from build123d import *

# Parameters (mm, degrees)
SKETCH3_W                      = 31.148374891
SKETCH3_H                      = 19.837641971
BOSS_EXTRUDE1_DEPTH            = 6.35
SKETCH4_R                      = 3.175
CUT_EXTRUDE1_DEPTH             = 9.525
SKETCH5_R                      = 3.175
CUT_EXTRUDE5_DEPTH             = 9.525
CUT_EXTRUDE5_DIRECTION_2_REACH = 33.299
SKETCH6_R                      = 3.175
CUT_EXTRUDE6_DEPTH             = 9.525
SKETCH8_W                      = 12.7
SKETCH8_H                      = 1.803641971
CUT_EXTRUDE7_DEPTH             = 38.470999417
SKETCH9_W                      = 1.905
SKETCH9_H                      = 18.034
BOSS_EXTRUDE2_DEPTH            = 4.7625
SKETCH11_W                     = 1.190625
SKETCH11_H                     = 1.906


with BuildPart() as part:
    # Sketch3 → Boss-Extrude1 (new, symmetric)
    with BuildSketch(Plane.XY):
        with Locations((15.574187446, -9.918820986)):
            Rectangle(SKETCH3_W, SKETCH3_H)
    extrude(amount=BOSS_EXTRUDE1_DEPTH, both=True)

    # Sketch4 → Cut-Extrude1 (cut)
    with BuildSketch(Plane.ZY):
        with Locations(Location((0, -6.35, 0), (0, 0, 270))):
            Circle(SKETCH4_R)
    cut_extrude1 = extrude(amount=-CUT_EXTRUDE1_DEPTH, mode=Mode.SUBTRACT)

    # Sketch5 → Cut-Extrude5 (cut)
    with BuildSketch(Plane(origin=(7.787093723, -19.837641971, 0), x_dir=(-0.8660254037844382, 0.500000000000001, 0), z_dir=(-0.500000000000001, -0.8660254037844382, 0))):
        with Locations(Location((0, 0, 0), (0, 0, 180))):
            Circle(SKETCH5_R)
    cut_extrude5 = extrude(amount=-CUT_EXTRUDE5_DEPTH, mode=Mode.SUBTRACT)

    # Sketch5 → Cut-Extrude5 direction 2 (cut, up to next)
    with BuildSketch(Plane(origin=(7.787093723, -19.837641971, 0), x_dir=(-0.8660254037844382, 0.500000000000001, 0), z_dir=(-0.500000000000001, -0.8660254037844382, 0)), mode=Mode.PRIVATE) as cut_extrude5_direction_2_sk1:
        with Locations(Location((0, 0, 0), (0, 0, 180))):
            Circle(SKETCH5_R)
    cut_extrude5_direction_2_tool1 = extrude(cut_extrude5_direction_2_sk1.sketch, amount=CUT_EXTRUDE5_DIRECTION_2_REACH, mode=Mode.PRIVATE) & part.part
    cut_extrude5_direction_2 = cut_extrude5_direction_2_tool1.solids().sort_by_distance((7.787094, -19.837642, 0))[0]
    add(cut_extrude5_direction_2, mode=Mode.SUBTRACT)

    # Sketch6 → Cut-Extrude6 (cut)
    with BuildSketch(Plane(origin=(0, 0, -6.35), x_dir=(-1, 0, 0), z_dir=(0, 0, -1))):
        with Locations((-15.574187445, -6.35)):
            Circle(SKETCH6_R)
    extrude(amount=-CUT_EXTRUDE6_DEPTH, mode=Mode.SUBTRACT)

    # Mirror1: Cut-Extrude1, Cut-Extrude5, Cut-Extrude5 direction 2 across plane
    add(cut_extrude1.mirror(Plane.ZY.offset(-15.574187445)), mode=Mode.SUBTRACT)
    add(cut_extrude5.mirror(Plane.ZY.offset(-15.574187445)), mode=Mode.SUBTRACT)
    add(cut_extrude5_direction_2.mirror(Plane.ZY.offset(-15.574187445)), mode=Mode.SUBTRACT)

    # Sketch8 → Cut-Extrude7 (cut, through all)
    with BuildSketch(Plane(origin=(31.148374891, 0, 0), x_dir=(0, 0, -1), z_dir=(1, 0, 0))):
        with Locations((0, -18.935820986)):
            Rectangle(SKETCH8_W, SKETCH8_H)
    extrude(amount=-CUT_EXTRUDE7_DEPTH, mode=Mode.SUBTRACT)

    # Sketch9 → Boss-Extrude2 (add)
    with BuildSketch(Plane(origin=(31.148374891, 0, 0), x_dir=(0, 0, -1), z_dir=(1, 0, 0))):
        with Locations((5.3975, -9.017)):
            Rectangle(SKETCH9_W, SKETCH9_H)
    boss_extrude2 = extrude(amount=BOSS_EXTRUDE2_DEPTH)

    # Sketch11 → 3/32 (0.09375) Diameter Hole1 (revolve, cut)
    with BuildSketch(Plane(origin=(32.297076923, -9.525, -4.445), x_dir=(0, -1, 0), z_dir=(1, 0, 0))):
        with Locations((0.5953125, 0.953)):
            Rectangle(SKETCH11_W, SKETCH11_H)
    f_3_32_0_09375_diameter_hole1 = revolve(axis=Axis((32.297076923, -9.525, 1.905), (0, 0, -1)), mode=Mode.SUBTRACT)

    # Mirror2: Boss-Extrude2, 3/32 (0.09375) Diameter Hole1 across plane
    add(boss_extrude2.mirror(Plane.ZY.offset(-15.574187445)))
    add(f_3_32_0_09375_diameter_hole1.mirror(Plane.ZY.offset(-15.574187445)), mode=Mode.SUBTRACT)


solid = part.part
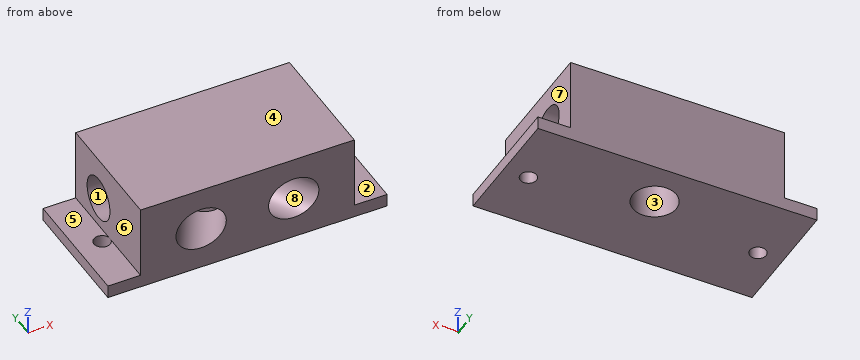
Geometry: final body of the model. Coordinates: model frame, mm. Face numbers are marked on the shaded views. A direction names the side the tool comes from. Give positions to 0.01 mm unless a question says otherwise; leave off trailing zeros. Loops run counter-clockwise (first coordinate to the right, second up) from the corner with the lowest first, then second, coordinate; pieces in that order, holes last. Notation, with made-up numbers: (-6, 40) - (30, 40) arc R14 ccw to (30, 66) - close; hole circle Ø10 at (72.25, 32). An arc over 180 degrees is marked (long way). Answer as CSV lines item,"result". Start each with the question number.
1. Section C-C, the plane x = 28.5. Return loops of the section in (y, z) (3 decimals), plus the area to 3 significant figures.
2. Reachability of the marked faces 1, 2, 3, 4 and 5 from +Z, -Z, +X, -X, +Y, -Y: full face, straight path, thin tool, end or side. Return the list, or none.
3. Section B-B, the plane z = 0. Return loops of the section in (x, y) (3 decimals).
4. Pin query (flat end, axial travel): P1, Ø1.4, axis at x = -1.5, y = -6, coming from the +Z side (3 decimals); P2, Ø5, axis at y = -6.5, z = 1, coming from the +X side; P3, Ø5, axis at y = -4.5, z = -3.5, coming from the +X side; P4, Ø5.5, axis at y = -6.35, z = 0, coming from the +X side. Return the tip coordinate at first contact, or that it passes through.
5. Ray query, L1, parallel to X at y = -6.5, z = -4.75; L2, parallel to X at y = -10.75, z = -1; L3, parallel to Y at x = 16.5, z = -1.5. Return the intervals inside material, ascending.
6. Draft query along X for the marked faces 6, 7 and 8. Return one class per face: released by +X, released by -X, zero draft, split by the parting line, or undercut.
Answers:
1,outline,"(-18.034, -6.35) - (0, -6.35) - (0, 6.35) - (-18.034, 6.35) - close; hole circle Ø6.35 at (-6.35, 0)"
1,area,"197 mm2"
2,face 1,"-X"
2,face 2,"+Z, +X, +Y, -Y"
2,face 3,"-Z"
2,face 4,"+Z, +X, -X, +Y, -Y"
2,face 5,"+Z, -X, +Y, -Y"
3,outline,"(0, -18.034) - (5.162, -18.034) - (9.8, -10.001) - (15.299, -13.176) - (12.495, -18.034) - (18.654, -18.034) - (15.849, -13.176) - (21.348, -10.001) - (25.986, -18.034) - (31.148, -18.034) - (31.148, -9.525) - (21.623, -9.525) - (21.623, -3.175) - (31.148, -3.175) - (31.148, 0) - (0, 0) - (0, -3.175) - (9.525, -3.175) - (9.525, -9.525) - (0, -9.525) - close; hole circle Ø6.35 at (15.574, -6.35)"
4,P1,"stops at z = -4.445"
4,P2,"stops at x = 31.15"
4,P3,"stops at x = 35.91"
4,P4,"stops at x = 21.62"
5,L1,"x = -4.76 to 12.4, 18.75 to 35.91"
5,L2,"x = 0 to 9.55, 11.1 to 20.05, 21.59 to 31.15"
5,L3,"y = -18.03 to -13.55, -12.8 to -9.39, -3.31 to 0"
6,face 6,"released by -X"
6,face 7,"released by +X"
6,face 8,"undercut"
